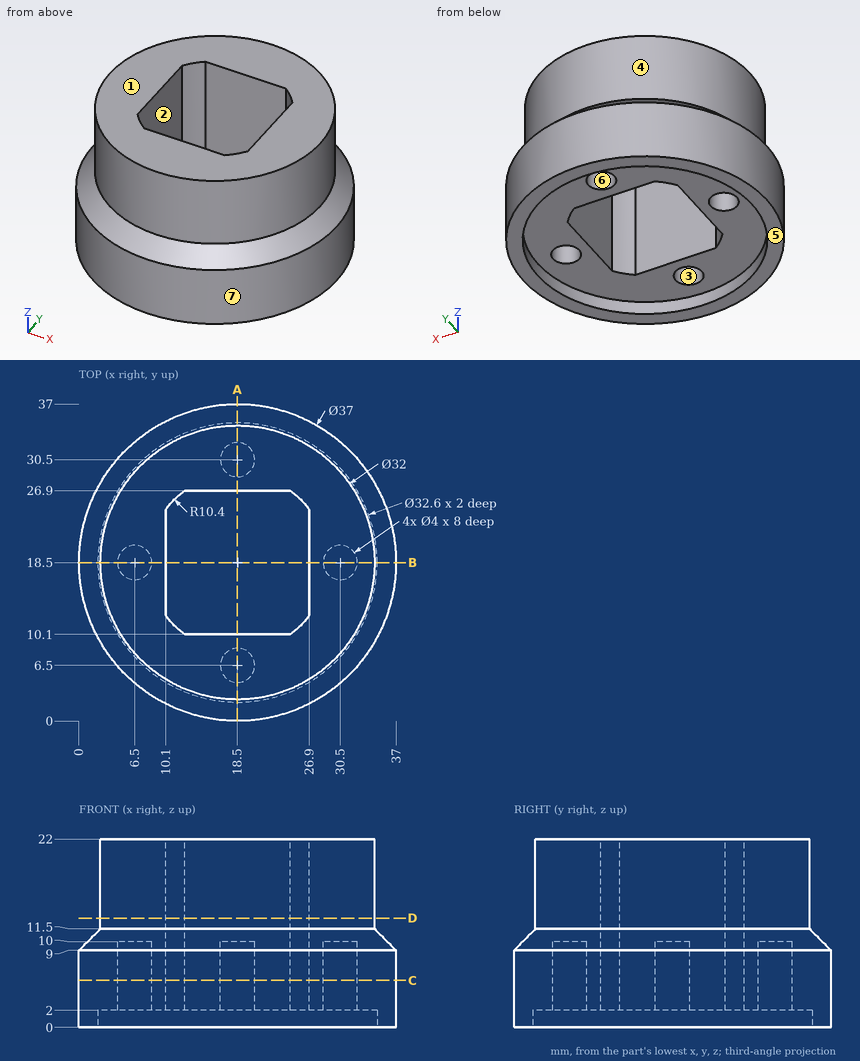
The figure shows three views and two pictorial views of one solid part (mm, origin at its lowest corner). Answer the questions. A direction names the side the tool comes from. Round coordinates to 2 decimals unless told otherwise and drop trailing zeros. Write each loop counter-clockwise with the first axis right and the second up, starting at its lowest first coordinate (ties: lowest second). Pieces come first, ordered by that corner, then holes. Notation, with made-up numbers: (31, -35) - (43, -35) arc R3 cw to (43, -31) - close; hole circle Ø5 at (52.25, 70). An arc over 180 degrees is marked (long way). One line per question, with ' | ' between items. Start each with the question number.
1. For the marked faces 1, 2, 3 and 4, determine the directions among +Z, -Z, +X, -X, +Y, -Y from which every point of the face is accessible in a straight line to the end or side of a thin tool.
2. Section C-C (z = 5.5) is taken. Determine the outline of the cut face in (x, y).
3. For a pull along Y with two mould halves and no side action, classify the marked faces 5, 6 and 7 as +Y half, -Y half, draft (parallel to the pull), parting line (faces both ways), or undercut.
4. Each of these flat-tipped pins is pushed along its axis until it touches: pin 1 (5 mm diameter, centred on x = 18.5, y = 30.5, fed in from -Z); pin 2 (1.2 mm diameter, centred on x = 6.5, y = 18, fed in from -Z); pin 3 (3.5 mm diameter, centred on x = 19.5, z = 13, fed in from +Y); pin 4 (2 mm diameter, centred on x = 13.5, y = 24.5, fed in from +Z). Where does it stop, or does it pass through?
5. Section A-A (x = 18.5) is taken. Determine the outline of the cut face in (y, z).
6. Section D-D (z = 12.75) is taken. Determine the outline of the cut face in (x, y), and give its area (3 significant figures).
7. Find the intervals of material crossed by probe 1 along Y at (x, z) = (18.5, 6.25); probe 2 along Y at (x, z) = (18.5, 1.2); probe 3 along Z at (x, y) = (31, 16), in increasing order. Write a range as [from, to].
Filled in:
1) face 1: +Z, +X, -X, +Y, -Y | face 2: +Z, -Z | face 3: -Z | face 4: +Z
2) outline: circle Ø37 at (18.5, 18.5); hole circle Ø4 at (6.5, 18.5); hole (10.1, 12.37) arc R10.4 ccw to (12.37, 10.1) - (24.63, 10.1) arc R10.4 ccw to (26.9, 12.37) - (26.9, 24.63) arc R10.4 ccw to (24.63, 26.9) - (12.37, 26.9) arc R10.4 ccw to (10.1, 24.63) - close; hole circle Ø4 at (18.5, 6.5); hole circle Ø4 at (18.5, 30.5); hole circle Ø4 at (30.5, 18.5)
3) face 5: draft | face 6: undercut | face 7: parting line
4) pin 1: z = 2 | pin 2: z = 10 | pin 3: y = 34.72 | pin 4: through
5) outline: (0, 0) - (2.2, 0) - (2.2, 2) - (4.5, 2) - (4.5, 10) - (8.5, 10) - (8.5, 2) - (10.1, 2) - (10.1, 22) - (2.5, 22) - (2.5, 11.5) - (0, 9) - close; (26.9, 2) - (28.5, 2) - (28.5, 10) - (32.5, 10) - (32.5, 2) - (34.8, 2) - (34.8, 0) - (37, 0) - (37, 9) - (34.5, 11.5) - (34.5, 22) - (26.9, 22) - close
6) outline: circle Ø32 at (18.5, 18.5); hole (10.1, 12.37) arc R10.4 ccw to (12.37, 10.1) - (24.63, 10.1) arc R10.4 ccw to (26.9, 12.37) - (26.9, 24.63) arc R10.4 ccw to (24.63, 26.9) - (12.37, 26.9) arc R10.4 ccw to (10.1, 24.63) - close | area: 531 mm²
7) probe 1: [0, 4.5], [8.5, 10.1], [26.9, 28.5], [32.5, 37] | probe 2: [0, 2.2], [34.8, 37] | probe 3: [2, 22]
